from build123d import *

# Parameters (mm, degrees)
SKETCH1_R           = 1.75
SKETCH1_R_2         = 1.5
BOSS_EXTRUDE1_DEPTH = 3.25
SKETCH2_W           = 9
SKETCH2_H           = 5
SKETCH2_R           = 1.5
BOSS_EXTRUDE2_DEPTH = 2
BOSS_EXTRUDE3_DEPTH = 2.5


with BuildPart() as part:
    # Sketch1 → Boss-Extrude1 (new body, symmetric)
    with BuildSketch(Plane(origin=(0, 0, 0), x_dir=(1, 0, 0), z_dir=(0, 1, 0))):
        Circle(SKETCH1_R)
        Circle(SKETCH1_R_2, mode=Mode.SUBTRACT)
    extrude(amount=BOSS_EXTRUDE1_DEPTH, both=True)

    # Sketch2 → Boss-Extrude2 (add)
    with BuildSketch(Plane(origin=(0, 3.25, 0), x_dir=(1, 0, 0), z_dir=(0, 1, 0))):
        Rectangle(SKETCH2_W, SKETCH2_H)
        Circle(SKETCH2_R, mode=Mode.SUBTRACT)
    boss_extrude2 = extrude(amount=-BOSS_EXTRUDE2_DEPTH)

    # Mirror1: Boss-Extrude2 across plane
    add(boss_extrude2.mirror(Plane.ZX))

    # Sketch3 → Boss-Extrude3 (add)
    with BuildSketch(Plane(origin=(0, -1.25, 0), x_dir=(1, 0, 0), z_dir=(0, 1, 0))):
        Polygon((0, 1.657655202), (-0.890187657, 1.657655202), (-0.890187657, 2.5), (0.95442496, 2.5), (0.95442496, 1.657655202), align=None)
        Polygon((0.95442496, -1.657655202), (0, -1.657655202), (-0.890187657, -1.657655202), (-0.890187657, -2.5), (0.95442496, -2.5), align=None)
    extrude(amount=BOSS_EXTRUDE3_DEPTH)


solid = part.part
Here's how the part is built. I have some questions about the finished solid (model axes, mm). A direction names the side the tool comes from. Round coordinates to 2 decimals unless told otherwise and drop trailing zeros. Write each loop counter-clockwise with the first axis right and the second up, starting at its lowest first coordinate (ties: lowest second). Pieces come first, ordered by that corner, then holes.
1. If we mould it in two halves opening along Z, with no side actions, what happens to faces 4 (the flat face through (0.954, 0, -2)), 5 (the cylindrical face through (-1.5, -0.05, -0.07)), 6 (the flat face through (0, 0, -2.5)), 7 (the flat face through (0, 0, 2.5))? For each: released by +Z, released by -Z, zero draft, split by the parting line, or undercut.
2. Suppose I cut it at C-C (y = 0.5). List the corners of the cut face in (x, z) for me, and give its area (3 significant figures).
3. Suppose I cut it at A-A (z = 0). List the corners of the cut face in (x, y) for me, and give its area (4 significant figures).
4. For faces 1 (the flat face through (4.5, -2, 0)), 2 (the flat face through (-0.89, 0, 2)), 3 (the flat face through (-0.89, 0, -2)), which set-ups out of +Z, -Z, +X, -X, +Y, -Y let a thin tool reach every point of the face, with its end or its side?
5. Will these pins go through, and if not, where does the flat tip stop? pin 1 Ø0.9 at (y, z) = (-0.5, 2) entering from +X; pin 2 Ø0.9 at (y, z) = (0.5, -2) entering from -X; pin 3 Ø2.5 at (x, z) = (0, 0) entering from +Y.
6. I need wall thicknesses on L1, parallel to Y at x = 3.5, z = 2; L2, parallel to Z at x = 0, y = 1.25; L3, parallel to X at y = -1.5, z = -0.05. Which ranges of each line are inside material? Lowest first, please.
7. Suppose I cut it at B-B (x = 0). List the corners of the cut face in (y, z) for me, and give its area (3 significant figures).
8. Suppose I cut it at D-D (x = -2.75). List the corners of the cut face in (y, z) for me, and give its area (3 significant figures).
Answer sheet:
1. face 4: zero draft
1. face 5: undercut
1. face 6: released by -Z
1. face 7: released by +Z
2. outline: (-0.89, -2.5) - (0.95, -2.5) - (0.95, -1.66) - (0.56, -1.66) arc R1.75 ccw to (0.56, 1.66) - (0.95, 1.66) - (0.95, 2.5) - (-0.89, 2.5) - (-0.89, 1.66) - (-0.56, 1.66) arc R1.75 ccw to (-0.56, -1.66) - (-0.89, -1.66) - close; hole circle Ø3 at (0, 0)
2. area: 5.52 mm2
3. outline: (-4.5, -3.25) - (-1.5, -3.25) - (-1.5, 3.25) - (-4.5, 3.25) - (-4.5, 1.25) - (-1.75, 1.25) - (-1.75, -1.25) - (-4.5, -1.25) - close; (1.5, -3.25) - (4.5, -3.25) - (4.5, -1.25) - (1.75, -1.25) - (1.75, 1.25) - (4.5, 1.25) - (4.5, 3.25) - (1.5, 3.25) - close
3. area: 25.25 mm2
4. face 1: +Z, -Z, +X, +Y, -Y
4. face 2: +Z, -X
4. face 3: -Z, -X
5. pin 1: stops at x = 0.95
5. pin 2: stops at x = -0.89
5. pin 3: passes through
6. L1: y = -3.25 to -1.25, 1.25 to 3.25
6. L2: z = -2.5 to -1.5, 1.5 to 2.5
6. L3: x = -4.5 to -1.5, 1.5 to 4.5
7. outline: (-3.25, -2.5) - (3.25, -2.5) - (3.25, -1.5) - (-3.25, -1.5) - close; (-3.25, 1.5) - (3.25, 1.5) - (3.25, 2.5) - (-3.25, 2.5) - close
7. area: 13.0 mm2
8. outline: (-3.25, -2.5) - (-1.25, -2.5) - (-1.25, 2.5) - (-3.25, 2.5) - close; (1.25, -2.5) - (3.25, -2.5) - (3.25, 2.5) - (1.25, 2.5) - close
8. area: 20.0 mm2
